Design review of the part built by this model. Coordinates are the model's own, in mm. A direction names the side the tool comes from. Give positions to 0.01 mm unless a question says otherwise; leave off trailing zeros. Use a Markdown table: item, result. Add a question column.
```python
from build123d import *

# Parameters (mm, degrees)
SKETCH1_R                       = 20
SKETCH1_R_2                     = 1
BOSS_EXTRUDE1_DEPTH             = 22.5
TAP_DRILL_FOR_M5X0_8_TAP1_D     = 4.2
TAP_DRILL_FOR_M5X0_8_TAP1_DEPTH = 5
TAP_DRILL_FOR_M5X0_8_TAP1_TIP   = 1.2618073
SKETCH4_W                       = 2.794
SKETCH4_H                       = 6.604
CUT_EXTRUDE1_DEPTH              = 20.5
CIRPATTERN1_COUNT               = 8
CUT_EXTRUDE3_START              = -6
SKETCH6_W                       = 4.62
SKETCH6_H                       = 8
SKETCH6_R                       = 2.1
CUT_EXTRUDE3_DEPTH              = 6
SKETCH7_R                       = 5.5
CUT_EXTRUDE4_DEPTH              = 1.8
SKETCH9_R                       = 3.014010562
CUT_EXTRUDE5_DEPTH              = 2
CHAMFER1_SIZE                   = 2
SKETCH8_R                       = 20
SKETCH8_R_2                     = 3
BOSS_EXTRUDE2_DEPTH             = 3
SKETCH5_R                       = 6
SKETCH5_R_2                     = 5
CUT_EXTRUDE2_DEPTH              = 0.909090909
FILLET3_R                       = 0.5
FILLET4_R                       = 2
CHAMFER2_SIZE                   = 0.1
CHAMFER2_SIZE2                  = 0.274747742


with BuildPart() as part:
    # Sketch1 → Boss-Extrude1 (new body)
    with BuildSketch(Plane.XY):
        with Locations(Location((-11.822558412, 14.529752947, 0), (0, 0, 180))):
            Circle(SKETCH1_R)
        with Locations(Location((-11.822558412, 14.529752947, 0), (0, 0, 180))):
            Circle(SKETCH1_R_2, mode=Mode.SUBTRACT)
    extrude(amount=BOSS_EXTRUDE1_DEPTH)

    # Tap Drill for M5x0.8 Tap1
    with Locations(Plane.XY.offset(22.5)):
        with Locations((-11.822558412, 14.529752947)):
            Hole(TAP_DRILL_FOR_M5X0_8_TAP1_D / 2, depth=TAP_DRILL_FOR_M5X0_8_TAP1_DEPTH)
            with Locations((0, 0, -(TAP_DRILL_FOR_M5X0_8_TAP1_DEPTH + TAP_DRILL_FOR_M5X0_8_TAP1_TIP / 2))):  # 118° drill point
                Cone(0, TAP_DRILL_FOR_M5X0_8_TAP1_D / 2, TAP_DRILL_FOR_M5X0_8_TAP1_TIP, mode=Mode.SUBTRACT)

    # Sketch4 → Cut-Extrude1 (cut)
    with BuildSketch(Plane.XY.offset(22.5)):
        with Locations((4.780441588, 14.531752947)):
            Rectangle(SKETCH4_W, SKETCH4_H)
    cut_extrude1 = extrude(amount=-CUT_EXTRUDE1_DEPTH, mode=Mode.SUBTRACT)

    # CirPattern1: Cut-Extrude1 ×8 about axis
    cirpattern1_axis = Axis((-11.822558412, 14.529752947, 0), (0, 0, 1))
    for i in range(1, CIRPATTERN1_COUNT):
        add(cut_extrude1.rotate(cirpattern1_axis, i * 360 / CIRPATTERN1_COUNT), mode=Mode.SUBTRACT)

    # Sketch6 → Cut-Extrude3 (cut)
    # profile 1 of 4: a face of its own
    with BuildSketch(Plane.XY.offset(22.5).offset(CUT_EXTRUDE3_START)):
        Polygon((-16.444354251, 14.529752947), (-14.132558412, 18.529752947), (-14.132558412, 10.529752947), align=None)
    # profile 2 of 4: a face of its own
    with BuildSketch(Plane.XY.offset(22.5).offset(CUT_EXTRUDE3_START)):
        Polygon((-7.200762573, 14.529752947), (-9.512558412, 10.529752947), (-9.512558412, 18.529752947), align=None)
    # profile 3 of 4: a face of its own
    with BuildSketch(Plane.XY.offset(22.5).offset(CUT_EXTRUDE3_START)):
        with Locations((-11.822558412, 14.529752947)):
            Rectangle(SKETCH6_W, SKETCH6_H)
        with Locations((-11.822558412, 14.529752947)):
            Circle(SKETCH6_R, mode=Mode.SUBTRACT)
    # profile 4 of 4: a face of its own
    with BuildSketch(Plane.XY.offset(22.5).offset(CUT_EXTRUDE3_START)):
        with Locations((-11.822558412, 14.529752947)):
            Circle(SKETCH6_R)
    extrude(amount=CUT_EXTRUDE3_DEPTH, mode=Mode.SUBTRACT)

    # Sketch7 → Cut-Extrude4 (cut)
    with BuildSketch(Plane.XY.offset(22.5)):
        with Locations((-11.822558412, 14.529752947)):
            Circle(SKETCH7_R)
    extrude(amount=-CUT_EXTRUDE4_DEPTH, mode=Mode.SUBTRACT)

    # Sketch9 → Cut-Extrude5 (cut)
    with BuildSketch(Plane.XY.offset(16.5)):
        with Locations((-11.822558412, 14.529752947)):
            Circle(SKETCH9_R)
    extrude(amount=-CUT_EXTRUDE5_DEPTH, mode=Mode.SUBTRACT)

    # Chamfer1
    chamfer1_edges = [part.edges().sort_by_distance(p)[0] for p in [
        (-14.836568974, 14.529752947, 14.5),
    ]]
    chamfer(chamfer1_edges, length=CHAMFER1_SIZE - 0.0001)  # a hair under: the kernel refuses the full size

    # Sketch8 → Boss-Extrude2 (add)
    with BuildSketch(Plane.XY.offset(22.5)):
        with Locations(Location((-11.822558412, 14.529752947, 0), (0, 0, 180))):
            Circle(SKETCH8_R)
        with Locations((-11.822558412, 14.529752947)):
            Circle(SKETCH8_R_2, mode=Mode.SUBTRACT)
    extrude(amount=BOSS_EXTRUDE2_DEPTH)

    # Sketch5 → Cut-Extrude2 (cut)
    with BuildSketch(Plane(origin=(0, 0, 0), x_dir=(-1, 0, 0), z_dir=(0, 0, -1))):
        with Locations((11.822558412, 14.529752947)):
            Circle(SKETCH5_R)
        with Locations((11.822558412, 14.529752947)):
            Circle(SKETCH5_R_2, mode=Mode.SUBTRACT)
    extrude(amount=-CUT_EXTRUDE2_DEPTH, mode=Mode.SUBTRACT)

    # Fillet3
    fillet3_edges = [part.edges().sort_by_distance(p)[0] for p in [
        (-5.822558412, 14.529752947, 0.909090909),
        (-6.822558412, 14.529752947, 0.909090909),
    ]]
    fillet(fillet3_edges, radius=FILLET3_R - 0.0001)  # a hair under: the kernel refuses the full size

    # Fillet4
    fillet4_edges = [part.edges().sort_by_distance(p)[0] for p in [
        (8.177441588, 14.529752947, 25.5),
    ]]
    fillet(fillet4_edges, radius=FILLET4_R)

    # Chamfer2
    chamfer2_edges = [part.edges().sort_by_distance(p)[0] for p in [
        (8.177441588, 14.529752947, 0),
    ]]
    chamfer2_side = [part.faces().sort_by_distance(p)[0] for p in [
        (7.611756163, 14.529752947, 0),
    ]]
    chamfer(chamfer2_edges, length=CHAMFER2_SIZE, length2=CHAMFER2_SIZE2, reference=chamfer2_side[0])


solid = part.part
```
1) Insertion check: pin 1 (5.5 mm diameter, centred on x = -13, z = 8.5, fed in from -Y); pin 2 (1.4 mm diameter, centred on y = 30.5, z = 8.5, fed in from -X); pin 3 (3 mm diameter, centred on y = 31.5, z = 8.5, fed in from +X). Each pin has a flat end and moves straight along its axis. Give the tip position at first contact, or say it passes through.
2) Machinability: for faces 1 (the flat face through (-12, 31, 2)), 2 (the cylindrical face through (-10.522, 8.672, 0.202)), which of the approach directions +Z, -Z, +X, -X, +Y, -Y give a long, thin tool a straight path to every point of the face, cutting with its end or side? Answer none if there is none.
3) Add section A-A (z = 7.25). Give the number of separate pieces and of enclosed holes in the cut face, then the cut area to 3 significant figures.
4) For L1, parallel to X at y = 24.5, z = 5.5; L2, parallel to Y at x = 0, z = 19.25; L3, parallel to X at y = 24, z = 11, list the stretches that pass through material, from the lowest coordinate up. Write a range as [from, to].
Worked answers:
| question | item | result |
|---|---|---|
| 1 | pin 1 | y = -5.47 |
| 1 | pin 2 | x = -24.74 |
| 1 | pin 3 | x = 0.85 |
| 2 | face 1 | none |
| 2 | face 2 | -Z |
| 3 | separate pieces | 1 |
| 3 | enclosed holes | 9 |
| 3 | area | 1,110 mm^2 |
| 4 | L1 | [-29.16, -26.47], [-23.36, -0.29], [2.81, 5.52] |
| 4 | L2 | [-1.6, 0.9], [4.85, 24.21], [28.16, 30.66] |
| 4 | L3 | [-29.44, -25.97], [-23.86, 0.21], [2.31, 5.79] |
